from build123d import *

# Parameters (mm, degrees)
BOSS_EXTRUDE3_DEPTH = 10


with BuildPart() as part:
    # Sketch1 → Boss-Extrude3 (new body)
    with BuildSketch(Plane.XY):
        with BuildLine():
            Line((19.582862725, 14.770272681), (30.960060849, 21.33890108))
            ThreePointArc((30.960060849, 21.33890108), (31.673214627, 23.712775149), (33.366924266, 25.522530399))
            ThreePointArc((33.366924266, 25.522530399), (21.00447091, 36.380810803), (5.419697562, 41.65786926))
            ThreePointArc((5.419697562, 41.65786926), (4.69925836, 39.286196061), (3, 37.481649738))
            Line((3, 37.481649738), (3, 23.393619776))
            Line((3, 23.393619776), (0, 24.838343632))
            Line((0, 24.838343632), (-3, 23.393619776))
            Line((-3, 23.393619776), (-3, 37.481649738))
            ThreePointArc((-3, 37.481649738), (-4.69925836, 39.286196061), (-5.419697562, 41.65786926))
            ThreePointArc((-5.419697562, 41.65786926), (-21.00447091, 36.380810803), (-33.366924266, 25.522530399))
            ThreePointArc((-33.366924266, 25.522530399), (-31.673214627, 23.712775149), (-30.960060849, 21.33890108))
            Line((-30.960060849, 21.33890108), (-19.582862725, 14.770272681))
            Line((-19.582862725, 14.770272681), (-20.980061971, 8.648742811))
            Line((-20.980061971, 8.648742811), (-33.960060849, 16.142748658))
            ThreePointArc((-33.960060849, 16.142748658), (-36.372472987, 15.573420912), (-38.786621827, 16.135338861))
            ThreePointArc((-38.786621827, 16.135338861), (-42.008941821, 0), (-38.786621827, -16.135338861))
            ThreePointArc((-38.786621827, -16.135338861), (-36.372472987, -15.573420912), (-33.960060849, -16.142748658))
            Line((-33.960060849, -16.142748658), (-21.490919097, -8.943686311))
            Line((-21.490919097, -8.943686311), (-17.707725135, -13.687661489))
            Line((-17.707725135, -13.687661489), (-30.960060849, -21.33890108))
            ThreePointArc((-30.960060849, -21.33890108), (-31.673214627, -23.712775149), (-33.366924266, -25.522530399))
            ThreePointArc((-33.366924266, -25.522530399), (-21.00447091, -36.380810803), (-5.419697562, -41.65786926))
            ThreePointArc((-5.419697562, -41.65786926), (-4.69925836, -39.286196061), (-3, -37.481649738))
            Line((-3, -37.481649738), (-3, -22.378574343))
            Line((-3, -22.378574343), (3, -22.378574343))
            Line((3, -22.378574343), (3, -37.481649738))
            ThreePointArc((3, -37.481649738), (4.69925836, -39.286196061), (5.419697562, -41.65786926))
            ThreePointArc((5.419697562, -41.65786926), (21.00447091, -36.380810803), (33.366924266, -25.522530399))
            ThreePointArc((33.366924266, -25.522530399), (31.673214627, -23.712775149), (30.960060849, -21.33890108))
            Line((30.960060849, -21.33890108), (17.707725135, -13.687661489))
            Line((17.707725135, -13.687661489), (21.490919097, -8.943686311))
            Line((21.490919097, -8.943686311), (33.960060849, -16.142748658))
            ThreePointArc((33.960060849, -16.142748658), (36.372472987, -15.573420912), (38.786621827, -16.135338861))
            ThreePointArc((38.786621827, -16.135338861), (42.008941821, 0), (38.786621827, 16.135338861))
            ThreePointArc((38.786621827, 16.135338861), (36.372472987, 15.573420912), (33.960060849, 16.142748658))
            Line((33.960060849, 16.142748658), (20.980061971, 8.648742811))
            Line((20.980061971, 8.648742811), (19.582862725, 14.770272681))
        make_face()
    extrude(amount=BOSS_EXTRUDE3_DEPTH)


solid = part.part
Read the model definition and answer for the solid it produces. Units are mm, in the model's axes. A direction names the side the tool comes from. Round coordinates to 2 decimals unless told otherwise and drop trailing zeros. Write each loop counter-clockwise with the first axis right and the second up, starting at its lowest first coordinate (ties: lowest second). Pieces come first, ordered by that corner, then holes. Notation, with made-up numbers: (31.5, 27) - (75.5, 27) arc R29 cw to (75.5, 64) - close; hole circle Ø10 at (43, -25). An arc over 180 degrees is marked (long way). One line per question, with ' | ' between items. Start each with the question number.
1. Section B-B (x = -22.5) is taken. Determine the outline of the cut face in (y, z), and give its area (3 significant figures).
2. Section D-D (x = -14) is taken. Determine the outline of the cut face in (y, z), and give its area (3 significant figures).
3. For a pull along Y with two mould halves and no side action, classify faces 4 (the face through (3, -30, 5)), 5 (the face through (19.57, -11.35, 4.93)), 6 (the face through (0, -22.379, 5)), 7 (the face through (-20.272, 11.752, 4.93)) as +Y half, -Y half, draft (parallel to the pull), parting line (faces both ways), or undercut.
4. Find the intervals of material crossed by probe 1 along Y at (x, z) = (-28.5, 4); probe 2 along Y at (x, z) = (-25.5, 5.75); probe 3 along X at (y, z) = (-12.5, 2.5), in increasing order. Write a range as [from, to].
5. Section A-A (y = 27.5) is taken. Determine the outline of the cut face in (x, z).
6. Each of these flat-tipped pins is pushed along its axis until it touches: pin 1 (1 mm diameter, centred on x = 8.5, z = 8.5, fed in from +Y); pin 2 (4 mm diameter, centred on x = -24.5, z = 4, fed in from -Y); pin 3 (1.5 mm diameter, centred on y = 33, z = 6, fed in from -X); pin 4 (2 mm diameter, centred on x = 6, y = 8.5, fed in from -Z). Where does it stop, or does it pass through?
7. For faces 1 (the face through (25.192, 18.009, 4.93)), 2 (the face through (31.69, -23.74, 4.93)), 3 (the face through (-4.72, -39.32, 4.93)), determine the directions among +Z, -Z, +X, -X, +Y, -Y from which every point of the face is accessible in a straight line to the end or side of a thin tool.
8. Section C-C (y = -30) is taken. Determine the outline of the cut face in (x, z).
Filled in:
1) outline: (-35.48, 0) - (-16.45, 0) - (-16.45, 10) - (-35.48, 10) - close; (-9.53, 0) - (9.53, 0) - (9.53, 10) - (-9.53, 10) - close; (16.45, 0) - (35.48, 0) - (35.48, 10) - (16.45, 10) - close | area: 571 mm²
2) outline: (-39.61, 0) - (39.61, 0) - (39.61, 10) - (-39.61, 10) - close | area: 792 mm²
3) face 4: draft | face 5: undercut | face 6: -Y half | face 7: undercut
4) probe 1: [-30.86, -19.92], [-12.99, 12.99], [19.92, 30.86] | probe 2: [-33.38, -18.19], [-11.26, 11.26], [18.19, 33.38] | probe 3: [-40.11, -27.65], [-18.65, 18.65], [27.65, 40.11]
5) outline: (-31.76, 0) - (-3, 0) - (-3, 10) - (-31.76, 10) - close; (3, 0) - (31.76, 0) - (31.76, 10) - (3, 10) - close
6) pin 1: y = 41.24 | pin 2: y = -35.48 | pin 3: x = -26.92 | pin 4: z = 0
7) face 1: +Z, -Z | face 2: +Z, -Z, +X | face 3: +Z, -Z, -Y
8) outline: (-29.41, 0) - (-3, 0) - (-3, 10) - (-29.41, 10) - close; (3, 0) - (29.41, 0) - (29.41, 10) - (3, 10) - close
